Can you work these out from the model? Positions are in its coordinate system, mm. A direction names the side the tool comes from. Round coordinates to 2 decimals unless told otherwise and drop trailing zeros. Order: outer loops, then holes, each group sorted by start corner. A loop starts at its lowest first (then second) coordinate and runs counter-clockwise, first axis right, second up.
Q1. We'd pull the mould along X, two halves only. Please class faces 1 (the face through (-59, -65.215, 7)), 2 (the face through (-88.83, -58.66, 4.38)), 3 (the face through (-21.04, -63.074, 7.28)): pulls with the +X half, pulls with the -X half, needs draft (parallel to the pull), parting line crosses it, or undercut.
Q2. Will these pins go through, and if not, where does the flat tip stop? P1, Ø1.5, axis at y = -50.5, z = 4.5, coming from the -X side; P2, Ø5, axis at y = -51, z = 4.5, coming from the -X side; P3, Ø1, axis at x = -45, z = 7.5, coming from the +Y side; P4, Ø1.5, axis at y = -58.5, z = 3, coming from the +X side.
Q3. For faces 4 (the face through (-33.76, -8.16, 2.82)), 5 (the face through (-26.12, -33.46, 7.28)), 6 (the face through (-55, -53.785, 7)), which set-ups out of +Z, -Z, +X, -X, +Y, -Y let a thin tool reach every point of the face, with its end or its side?
Q4. If we section it at A-A (z = 3.75): Please give me the cut outline in (x, y) (3 decimals).
Q5. If I drill on line 1 (Z direction, x = -61, y = -59.5) (3 decimals); line 2 (Y direction, x = -50, z = 7) (3 decimals); line 3 (Y direction, x = -41.5, z = 1.75), over which ranges is the centre line in solid material (lowest first)?
Q6. If we section it at B-B (y = -59.5): Please give me the cut outline in (x, z) (3 decimals).
Q7. If we section it at C-C (x = -66): Please give me the cut outline in (y, z) (3 decimals).
from build123d import *

# Parameters (mm, degrees)
SKETCH1_R             = 4.445
SKETCH1_R_2           = 2.8
BOSS_EXTRUDE1_DEPTH   = 5.715
BOSS_EXTRUDE1_2_DEPTH = 5.715
BOSS_EXTRUDE1_3_DEPTH = 5.715
SKETCH2_R             = 4.445
SKETCH2_R_2           = 2.8
BOSS_EXTRUDE5_DEPTH   = 3.175
SKETCH2_3_R           = 4.445
SKETCH2_3_R_2         = 2.8
BOSS_EXTRUDE6_DEPTH   = 3.175
CUT_EXTRUDE1_DEPTH    = 5.08
SKETCH4_R             = 1.75
CUT_EXTRUDE2_DEPTH    = 118.202447393


with BuildPart() as part:
    # Sketch1 → Boss-Extrude1 (new body)
    with BuildSketch(Plane.XY):
        with Locations((-91.5, -59.5)):
            Circle(SKETCH1_R)
        with Locations((-91.5, -59.5)):
            Circle(SKETCH1_R_2, mode=Mode.SUBTRACT)
    extrude(amount=BOSS_EXTRUDE1_DEPTH)



with BuildPart() as body_2:
    # Sketch1 → Boss-Extrude1 2 (new body)
    with BuildSketch(Plane.XY):
        with Locations((-25.5, -59.5)):
            Circle(SKETCH1_R)
        with Locations((-25.5, -59.5)):
            Circle(SKETCH1_R_2, mode=Mode.SUBTRACT)
    extrude(amount=BOSS_EXTRUDE1_2_DEPTH)


with BuildPart() as body_3:
    # Sketch1 → Boss-Extrude1 3 (new body)
    with BuildSketch(Plane.XY):
        with Locations((-38, -9.5)):
            Circle(SKETCH1_R)
        with Locations((-38, -9.5)):
            Circle(SKETCH1_R_2, mode=Mode.SUBTRACT)
    extrude(amount=BOSS_EXTRUDE1_3_DEPTH)


with BuildPart() as part_1:
    add(part.part)

    add(body_3.part)  # Boss-Extrude5 merges body 3
    # Sketch2 → Boss-Extrude5 (add)
    with BuildSketch(Plane.XY.offset(5.715)):
        with BuildLine():
            Line((-19.955635612, -58.113908903), (-32.455635612, -8.113908903))
            ThreePointArc((-32.455635612, -8.113908903), (-36.381608185, -4.018938704), (-41.902228623, -5.324615374))
            Line((-41.902228623, -5.324615374), (-95.402228623, -55.324615374))
            ThreePointArc((-95.402228623, -55.324615374), (-96.816180402, -61.597486813), (-91.5, -65.215))
            Line((-91.5, -65.215), (-25.5, -65.215))
            ThreePointArc((-25.5, -65.215), (-20.995405922, -63.017080777), (-19.955635612, -58.113908903))
        make_face()
        with Locations((-25.5, -59.5)):
            Circle(SKETCH2_R, mode=Mode.SUBTRACT)
        Polygon((-77.015059827, -53.785), (-41.189982364, -20.303619193), (-32.819637163, -53.785), align=None, mode=Mode.SUBTRACT)
        with Locations((-91.5, -59.5)):
            Circle(SKETCH2_R_2, mode=Mode.SUBTRACT)
        with Locations(Location((-38, -9.5, 0), (0, 0, 180))):
            Circle(SKETCH2_R_2, mode=Mode.SUBTRACT)
    extrude(amount=BOSS_EXTRUDE5_DEPTH)


    add(body_2.part)  # Boss-Extrude6 merges body 2
    # Sketch2<3> → Boss-Extrude6 (add)
    with BuildSketch(Plane.XY.offset(5.715)):
        with Locations((-25.5, -59.5)):
            Circle(SKETCH2_3_R)
        with Locations((-25.5, -59.5)):
            Circle(SKETCH2_3_R_2, mode=Mode.SUBTRACT)
    extrude(amount=BOSS_EXTRUDE6_DEPTH)

    # Sketch3 → Cut-Extrude1 (cut)
    with BuildSketch(Plane.XY.offset(8.89)):
        with BuildLine():
            ThreePointArc((-75.8, -59.5), (-77.55, -57.75), (-79.3, -59.5))
            Line((-79.3, -59.5), (-75.8, -59.5))
        make_face()
        with BuildLine():
            Line((-75.8, -59.5), (-79.3, -59.5))
            ThreePointArc((-79.3, -59.5), (-77.55, -61.25), (-75.8, -59.5))
        make_face()
        with BuildLine():
            ThreePointArc((-37.7, -59.5), (-39.45, -57.75), (-41.2, -59.5))
            Line((-41.2, -59.5), (-37.7, -59.5))
        make_face()
        with BuildLine():
            Line((-37.7, -59.5), (-41.2, -59.5))
            ThreePointArc((-41.2, -59.5), (-39.45, -61.25), (-37.7, -59.5))
        make_face()
    extrude(amount=-CUT_EXTRUDE1_DEPTH, mode=Mode.SUBTRACT)

    # Sketch4 → Cut-Extrude2 (cut, through all)
    with BuildSketch(Plane(origin=(0, 0, 5.715), x_dir=(-1, 0, 0), z_dir=(0, 0, -1))):
        with Locations((52.503366943, -23.745857138)):
            Circle(SKETCH4_R)
    extrude(amount=-CUT_EXTRUDE2_DEPTH, mode=Mode.SUBTRACT)


solid = part_1.part
Solution:
1. face 1: needs draft
1. face 2: undercut
1. face 3: pulls with the +X half
2. P1: passes through
2. P2: stops at x = -93.11
2. P3: stops at y = -7.75
2. P4: stops at x = -21.06
3. face 4: -Z
3. face 5: +Z, -Z, +X, +Y
3. face 6: +Z, -Z
4. outline: circle Ø8.89 at (-91.5, -59.5); circle Ø8.89 at (-38, -9.5); circle Ø8.89 at (-25.5, -59.5); hole circle Ø5.6 at (-91.5, -59.5); hole circle Ø5.6 at (-38, -9.5); hole circle Ø5.6 at (-25.5, -59.5)
5. line 1: z = 5.715 to 8.89
5. line 2: y = -65.215 to -53.785, -28.537 to -12.893
5. line 3: y = -12.24 to -6.76
6. outline: (-97.215, 5.715) - (-95.945, 5.715) - (-95.945, 0) - (-94.3, 0) - (-94.3, 8.89) - (-97.215, 8.89) - close; (-88.7, 0) - (-87.055, 0) - (-87.055, 5.715) - (-79.3, 5.715) - (-79.3, 8.89) - (-88.7, 8.89) - close; (-75.8, 5.715) - (-41.2, 5.715) - (-41.2, 8.89) - (-75.8, 8.89) - close; (-37.7, 5.715) - (-29.945, 5.715) - (-29.945, 0) - (-28.3, 0) - (-28.3, 8.89) - (-37.7, 8.89) - close; (-22.7, 0) - (-21.055, 0) - (-21.055, 5.715) - (-19.785, 5.715) - (-19.785, 8.89) - (-22.7, 8.89) - close
7. outline: (-65.215, 5.715) - (-53.785, 5.715) - (-53.785, 8.89) - (-65.215, 8.89) - close; (-43.491, 5.715) - (-27.846, 5.715) - (-27.846, 8.89) - (-43.491, 8.89) - close
